from build123d import *

# Parameters (mm, degrees)
SKETCH1_W               = 40
SKETCH1_H               = 120
SKETCH3_R               = 3.821172455
BOSS_EXTRUDE1_DEPTH     = 15
SKETCH5_R               = 27.5
BOSS_EXTRUDE2_DEPTH     = 60
SKETCH4_R               = 22.5
CUT_EXTRUDE2_DEPTH      = 20
SKETCH2_R               = 20
CUT_EXTRUDE3_DEPTH      = 61.0000001
CUT_EXTRUDE3_DEPTH_BACK = 61.0000001


with BuildPart() as part:
    # Sketch1 → Base-Revolve (revolve)
    with BuildSketch(Plane.XY):
        with Locations((20, -50)):
            Rectangle(SKETCH1_W, SKETCH1_H)
    revolve(axis=Axis((0, 300, 0), (0, -1, 0)))

    # Sketch3 → Boss-Extrude1 (add, symmetric)
    with BuildSketch(Plane.XY):
        with BuildLine():
            Line((30, -5), (60, -20))
            ThreePointArc((60, -20), (63.090169944, -25), (60, -30))
            Line((60, -30), (30, -45))
            Line((30, -45), (30, -5))
        make_face()
        with Locations((57.5, -25)):
            Circle(SKETCH3_R, mode=Mode.SUBTRACT)
    boss_extrude1 = extrude(amount=BOSS_EXTRUDE1_DEPTH, both=True)

    # Mirror1: Boss-Extrude1 across plane
    add(boss_extrude1.mirror(Plane(origin=(0, 0, 0), x_dir=(0, 0, 1), z_dir=(1, 0, 0))))

    # Sketch5 → Boss-Extrude2 (add, symmetric)
    with BuildSketch(Plane.XY):
        with Locations((0, -70)):
            Circle(SKETCH5_R)
    extrude(amount=BOSS_EXTRUDE2_DEPTH, both=True)

    # Sketch4 → Cut-Extrude2 (cut)
    with BuildSketch(Plane(origin=(0, 10, 0), x_dir=(-1, 0, 0), z_dir=(0, 1, 0))):
        Circle(SKETCH4_R)
    extrude(amount=-CUT_EXTRUDE2_DEPTH, mode=Mode.SUBTRACT)

    # Sketch2 → Cut-Extrude3 (cut, two sides)
    with BuildSketch(Plane.XY) as cut_extrude3_sk:
        with Locations((0, -70)):
            Circle(SKETCH2_R)
    extrude(amount=CUT_EXTRUDE3_DEPTH, mode=Mode.SUBTRACT)
    extrude(cut_extrude3_sk.sketch, amount=-CUT_EXTRUDE3_DEPTH_BACK, mode=Mode.SUBTRACT)


solid = part.part
Can you work these out from the model? Positions are in its coordinate system, mm. A direction names the side the tool comes from. Coordinates: 2 decimals unless noted, no trailing zeros. Loops run counter-clockwise (first coordinate to the right, second up) from the corner with the lowest first, then second, coordinate; pieces in that order, holes last. Notation, with made-up numbers: (47.25, 83.25) - (103.25, 83.25) arc R13 cw to (103.25, 97.25) - close; hole circle Ø6 at (5.25, -20). An arc over 180 degrees is marked (long way). Put each result on its own line as item: value. Start each with the question number.
Item 1: If I drill on line 1 along X through (y, z) = (-24.5, -2); line 2 along Y through (x, z) = (0, 25); line 3 along X through (y, z) = (-21.5, 2.5), over which ranges is the centre line in solid material (lowest first)?
Item 2: Suppose I cut it at D-D (z = 0). Please give me the cut outline in (x, y), and give its area (3 significant figures).
Item 3: Which directions (+Z, -Z, +X, -X, +Y, -Y) give clear straight access to the entire face, cutting with the end or side of a thin tool? Please do faces 4 (the face through (47, -25, 15)), 5 (the face through (26.23, -61.74, 48.18)), 6 (the face through (-47, -25, -15)).
Item 4: For pin 1 (12 mm diameter, centred on x = -34.5, y = -72, fed in from -Z); pin 2 (13 mm diameter, centred on x = 45.5, y = -27.5, fed in from +Z); pin 3 (4 mm diameter, centred on x = 35.5, y = -41.5, fed in from -Z); pin 4 (8 mm diameter, centred on x = -49, z = -20, fed in from +Y), each with a flat end and sliding along its axis, tell me the tip position at first contact or that it passes through.
Item 5: Suppose I cut it at B-B (x = 0). Please give me the cut outline in (y, z), and give its area (3 significant figures).
Item 6: Suppose I cut it at C-C (z = -37.5). Please give me the cut outline in (x, y), and give its area (3 significant figures).
Item 7: If we mould it in two halves opening along Y, with no side actions, what happens to faces 1 (the face through (-47, -25, 15)), 2 (the face through (48.7, -35.65, 0.21)), 3 (the face through (53.683, -24.832, -0.21))? For each: +Y half, -Y half, draft (parallel to the pull), parting line (faces both ways), or undercut.
Item 8: Suppose I cut it at A-A (y = -70). Please give me the cut outline in (x, z).
Here are the results:
1. line 1: -63.07 to -61.29, -53.71 to 53.71, 61.29 to 63.07
1. line 2: -110 to -90, -50 to 10
1. line 3: -61.86 to -59.03, -55.97 to 55.97, 59.03 to 61.86
2. outline: (-60, -30) - (-40, -40) - (-40, -110) - (40, -110) - (40, -40) - (60, -30) arc R5.59 ccw to (60, -20) - (40, -10) - (40, 10) - (22.5, 10) - (22.5, -10) - (-22.5, -10) - (-22.5, 10) - (-40, 10) - (-40, -10) - (-60, -20) arc R5.59 ccw to start; hole circle Ø7.64 at (-57.5, -25); hole circle Ø40 at (0, -70); hole circle Ø7.64 at (57.5, -25)
2. area: 8,200 mm²
3. face 4: +Z, +X, +Y, -Y
3. face 5: +Z
3. face 6: -Z, -X, +Y, -Y
4. pin 1: z = -28.07
4. pin 2: z = 15
4. pin 3: z = -21.86
4. pin 4: through
5. outline: (-110, -40) - (-97.5, -40) - (-97.5, -60) - (-90, -60) - (-90, 60) - (-97.5, 60) - (-97.5, 40) - (-110, 40) - close; (-50, -60) - (-42.5, -60) - (-42.5, -40) - (10, -40) - (10, -22.5) - (-10, -22.5) - (-10, 22.5) - (10, 22.5) - (10, 40) - (-42.5, 40) - (-42.5, 60) - (-50, 60) - close
5. area: 6,100 mm²
6. outline: (-13.92, -110) - (13.92, -110) - (13.92, -93.72) arc R27.5 ccw to (13.92, -46.28) - (13.92, 10) - (-13.92, 10) - (-13.92, -46.28) arc R27.5 ccw to (-13.92, -93.72) - close; hole circle Ø40 at (0, -70)
6. area: 3,000 mm²
7. face 1: draft
7. face 2: -Y half
7. face 3: undercut
8. outline: (-27.5, -60) - (-20, -60) - (-20, 60) - (-27.5, 60) - (-27.5, 29.05) arc R40 ccw to (-27.5, -29.05) - close; (20, -60) - (27.5, -60) - (27.5, -29.05) arc R40 ccw to (27.5, 29.05) - (27.5, 60) - (20, 60) - close
